Model file for the job. Use its own axes, mm. A direction names the side the tool comes from. Coordinates: 2 decimals unless noted, no trailing zeros. Write each loop counter-clockwise with the first axis right and the second up, starting at its lowest first coordinate (ties: lowest second). Pieces come first, ordered by that corner, then holes. Notation, with made-up numbers: M 14.5,8 L 39.5,8 A20 ccw 39.5,28 Z; hole C 60.25,36.25 d6. An arc over 180 degrees is marked long. Answer in a Markdown table with one row per item. Add a question column.
```python
from build123d import *

# Parameters (mm, degrees)
SKETCH1_R           = 1.5
BOSS_EXTRUDE1_DEPTH = 10
SKETCH2_R           = 14
CUT_EXTRUDE1_DEPTH  = 9.5
CUT_EXTRUDE2_START  = -10
CUT_EXTRUDE2_DEPTH  = 10
SKETCH4_R           = 1.5
BOSS_EXTRUDE2_DEPTH = 7.5
CUT_EXTRUDE3_START  = -7.5
CUT_EXTRUDE3_DEPTH  = 7.5


with BuildPart() as part:
    # Sketch1 → Boss-Extrude1 (new body)
    with BuildSketch(Plane(origin=(0, 0, 0), x_dir=(1, 0, 0), z_dir=(0, 1, 0))):
        with BuildLine():
            Line((-12, 15), (12, 15))
            ThreePointArc((12, 15), (14.121320344, 14.121320344), (15, 12))
            Line((15, 12), (15, -12))
            ThreePointArc((15, -12), (14.121320344, -14.121320344), (12, -15))
            Line((12, -15), (-12, -15))
            ThreePointArc((-12, -15), (-14.121320344, -14.121320344), (-15, -12))
            Line((-15, -12), (-15, 12))
            ThreePointArc((-15, 12), (-14.121320344, 14.121320344), (-12, 15))
        make_face()
        with Locations(Location((-12, -12, 0), (0, 0, 270))):
            Circle(SKETCH1_R, mode=Mode.SUBTRACT)
        with Locations(Location((-12, 12, 0), (0, 0, 270))):
            Circle(SKETCH1_R, mode=Mode.SUBTRACT)
        with Locations(Location((12, 12, 0), (0, 0, 270))):
            Circle(SKETCH1_R, mode=Mode.SUBTRACT)
        with Locations(Location((12, -12, 0), (0, 0, 270))):
            Circle(SKETCH1_R, mode=Mode.SUBTRACT)
    extrude(amount=BOSS_EXTRUDE1_DEPTH)

    # Sketch2 → Cut-Extrude1 (cut)
    with BuildSketch(Plane(origin=(0, 10, 0), x_dir=(1, 0, 0), z_dir=(0, 1, 0))):
        with Locations(Location((0, 0, 0), (0, 0, 270))):
            Circle(SKETCH2_R)
    extrude(amount=-CUT_EXTRUDE1_DEPTH, mode=Mode.SUBTRACT)

    # Sketch3 → Cut-Extrude2 (cut)
    with BuildSketch(Plane.XZ.offset(CUT_EXTRUDE2_START)):
        with BuildLine():
            Line((6.937196595, -2.850491783), (12.593386622, -6.116094618))
            ThreePointArc((12.593386622, -6.116094618), (12.124355653, 7), (1, 13.964240044))
            Line((1, 13.964240044), (1, 7.433034374))
            ThreePointArc((1, 7.433034374), (6.495190528, 3.75), (6.937196595, -2.850491783))
        make_face()
        with BuildLine():
            Line((5.937196595, -4.582542591), (11.593386622, -7.848145426))
            ThreePointArc((11.593386622, -7.848145426), (0, -14), (-11.593386622, -7.848145426))
            Line((-11.593386622, -7.848145426), (-5.937196595, -4.582542591))
            ThreePointArc((-5.937196595, -4.582542591), (0, -7.5), (5.937196595, -4.582542591))
        make_face()
        with BuildLine():
            Line((-1, 7.433034374), (-1, 13.964240044))
            ThreePointArc((-1, 13.964240044), (-12.124355653, 7), (-12.593386622, -6.116094618))
            Line((-12.593386622, -6.116094618), (-6.937196595, -2.850491783))
            ThreePointArc((-6.937196595, -2.850491783), (-6.495190528, 3.75), (-1, 7.433034374))
        make_face()
    extrude(amount=CUT_EXTRUDE2_DEPTH, mode=Mode.SUBTRACT)

    # Sketch4 → Boss-Extrude2 (add)
    with BuildSketch(Plane(origin=(0, 0.5, 0), x_dir=(1, 0, 0), z_dir=(0, 1, 0))):
        with Locations(Location((0, 0, 0), (0, 0, 270))):
            Circle(SKETCH4_R)
    extrude(amount=BOSS_EXTRUDE2_DEPTH)

    # Sketch5 → Cut-Extrude3 (cut)
    with BuildSketch(Plane(origin=(0, 10, 0), x_dir=(1, 0, 0), z_dir=(0, 1, 0)).offset(CUT_EXTRUDE3_START)):
        with BuildLine():
            Line((-6.213203436, 15), (-8.485281374, 12.727922061))
            Line((-8.485281374, 12.727922061), (-9.878679656, 14.121320344))
            ThreePointArc((-9.878679656, 14.121320344), (-10.851949703, 14.771638598), (-12, 15))
            Line((-12, 15), (-6.213203436, 15))
        make_face()
        with BuildLine():
            Line((-14.121320344, 9.878679656), (-12.727922061, 8.485281374))
            Line((-12.727922061, 8.485281374), (-15, 6.213203436))
            Line((-15, 6.213203436), (-15, 12))
            ThreePointArc((-15, 12), (-14.771638598, 10.851949703), (-14.121320344, 9.878679656))
        make_face()
        with BuildLine():
            Line((15, 6.213203436), (12.727922061, 8.485281374))
            Line((12.727922061, 8.485281374), (14.121320344, 9.878679656))
            ThreePointArc((14.121320344, 9.878679656), (14.771638598, 10.851949703), (15, 12))
            Line((15, 12), (15, 6.213203436))
        make_face()
        with BuildLine():
            Line((9.878679656, 14.121320344), (8.485281374, 12.727922061))
            Line((8.485281374, 12.727922061), (6.213203436, 15))
            Line((6.213203436, 15), (12, 15))
            ThreePointArc((12, 15), (10.851949703, 14.771638598), (9.878679656, 14.121320344))
        make_face()
        with BuildLine():
            Line((6.213203436, -15), (8.485281374, -12.727922061))
            Line((8.485281374, -12.727922061), (9.878679656, -14.121320344))
            ThreePointArc((9.878679656, -14.121320344), (10.851949703, -14.771638598), (12, -15))
            Line((12, -15), (6.213203436, -15))
        make_face()
        with BuildLine():
            Line((14.121320344, -9.878679656), (12.727922061, -8.485281374))
            Line((12.727922061, -8.485281374), (15, -6.213203436))
            Line((15, -6.213203436), (15, -12))
            ThreePointArc((15, -12), (14.771638598, -10.851949703), (14.121320344, -9.878679656))
        make_face()
        with BuildLine():
            Line((-15, -6.213203436), (-12.727922061, -8.485281374))
            Line((-12.727922061, -8.485281374), (-14.121320344, -9.878679656))
            ThreePointArc((-14.121320344, -9.878679656), (-14.771638598, -10.851949703), (-15, -12))
            Line((-15, -12), (-15, -6.213203436))
        make_face()
        with BuildLine():
            Line((-9.878679656, -14.121320344), (-8.485281374, -12.727922061))
            Line((-8.485281374, -12.727922061), (-6.213203436, -15))
            Line((-6.213203436, -15), (-12, -15))
            ThreePointArc((-12, -15), (-10.851949703, -14.771638598), (-9.878679656, -14.121320344))
        make_face()
    extrude(amount=CUT_EXTRUDE3_DEPTH, mode=Mode.SUBTRACT)


solid = part.part
```
1) Slice it at C-C (z = -9.25). Give the cut face in (x, y), then the cut area to 3 significant figures.
2) Drill centre lines: probe 1 along X at (y, z) = (7.25, 12); probe 2 along X at (y, z) = (0.75, -12.25); probe 3 along Z at (x, y) = (2.5, 5). Where is each one in solid material? Low to high.
3) Two-plate mould, pull along Z, no slides. Class faces 6 (the face through (14, 2.5, 8)), 7 (the face through (0, 4, 15)), 8 (the face through (0, 0, 0)), 9 (the face through (9.19, 6.2, -13.43)): released by +Z, released by -Z, zero draft, split by the parting line, or undercut.
4) Slice it at B-B (z = 0). Give the cut face in (x, y).
5) Which spindle directions (+Z, -Z, +X, -X, +Y, -Y) get a long thin tool onto all of the face, cutting with end or side? Do faces 1 (the face through (15, 4, 0)), 2 (the face through (9.17, 6.2, 13.41)), 3 (the face through (9, 2.5, -14)), 4 (the face through (8.726, 0.254, -6.192)), 5 (the face through (0, 4, -15)). Say none if no direction does.
6) Slice it at D-D (x = 2.75). Give the cut face in (y, z).
7) Slice it at A-A (y = 1.25). Give the cut face in (x, z), then the cut area to 3 significant figures.
8) Flat gauge pins, fed straight in: pin 1 Ø0.7 at (x, z) = (-14.5, 8.5) entering from +Y; pin 2 Ø6.5 at (x, z) = (-1, 8) entering from +Y; pin 3 Ø2.5 at (x, z) = (-12, -12) entering from +Y; pin 4 Ø1.5 at (x, z) = (0, -0.5) entering from +Y. Where does each tip first touch, or does it go through?
Ans:
| question | item | result |
|---|---|---|
| 1 | outline | M -15,0 L -10.51,0 L -10.51,10 L -13.49,10 L -13.49,2.5 L -15,2.5 Z; M 10.51,0 L 15,0 L 15,2.5 L 13.49,2.5 L 13.49,10 L 10.51,10 Z |
| 1 | area | 67.2 mm2 |
| 2 | probe 1 | x = -15 to -13.5, -10.5 to -7.21, 7.21 to 10.5, 13.5 to 15 |
| 2 | probe 2 | x = -14.99 to -13.48, -10.52 to -6.78, 6.78 to 10.52, 13.48 to 14.99 |
| 2 | probe 3 | z = -15 to -13.77, 13.77 to 15 |
| 3 | face 6 | undercut |
| 3 | face 7 | released by +Z |
| 3 | face 8 | zero draft |
| 3 | face 9 | released by -Z |
| 4 | outline | M -15,0 L -14,0 L -14,10 L -15,10 Z; M -7.5,0 L 7.5,0 L 7.5,0.5 L 1.5,0.5 L 1.5,8 L -1.5,8 L -1.5,0.5 L -7.5,0.5 Z; M 14,0 L 15,0 L 15,10 L 14,10 Z |
| 5 | face 1 | +Z, -Z, +X, +Y, -Y |
| 5 | face 2 | +Z, +Y |
| 5 | face 3 | -Z, +Y |
| 5 | face 4 | +Y, -Y |
| 5 | face 5 | -Z, +X, -X, +Y, -Y |
| 6 | outline | M 0,-15 L 10,-15 L 10,-13.73 L 0,-13.73 Z; M 0,-6.98 L 0.5,-6.98 L 0.5,6.98 L 0,6.98 Z; M 0,13.73 L 10,13.73 L 10,15 L 0,15 Z |
| 7 | outline | M -15,-12 A3 ccw -12,-15 L 12,-15 A3 ccw 15,-12 L 15,12 A3 ccw 12,15 L -12,15 A3 ccw -15,12 Z; C 0,0 d3; hole C 0,0 d28; hole C -12,-12 d3; hole C -12,12 d3; hole C 12,-12 d3; hole C 12,12 d3 |
| 7 | area | 255 mm2 |
| 8 | pin 1 | stops at y = 2.5 |
| 8 | pin 2 | stops at y = 0.5 |
| 8 | pin 3 | passes through |
| 8 | pin 4 | stops at y = 8 |
